Autodesk Inventor part; units mm, degrees
ref_plane "Work Plane1" through (0, 0, 0) normal (0, 0, 1) x (1, 0, 0)
ref_plane "Work Plane2" through (175.2488, -178.5172, -25.4) normal (0, 0, 1) x (0.3503, -0.9366, 0)
ref_plane "YZ Plane" through (0, 0, 0) normal (1, 0, 0) x (0, 1, 0)
ref_plane "Work Plane1" through (0, 0, 0) normal (0, 0, 1) x (1, 0, 0)
sketch "Sketch1" plane through (0, 0, 0) normal (0, 0, 1) x (1, 0, 0)
  circle A0 centre (0, 0) radius 12.7
  dimension "d0" = 25.4
extrude "Extrusion1" add sketch "Sketch1" against normal blind 50.8
sketch "Sketch2" plane through (0, 0, 0) normal (0, 0, 1) x (1, 0, 0)
  circle A0 centre (0, 0) radius 12.7
extrude "Extrusion2" add sketch "Sketch2" along normal blind 50.8
sketch "Sketch4" plane through (0, 0, 50.8) normal (0, 0, 1) x (1, 0, 0)
  circle A0 centre (0, 0) radius 38.1
  dimension "d6" = 76.2
extrude "Extrusion3" add sketch "Sketch4" along normal blind 25.4
ref_plane "Work Plane2" through (175.2488, -178.5172, -25.4) normal (0, 0, 1) x (0.3503, -0.9366, 0)
properties part number "clutch02-releaseMechanism" material "PET Plastic"
Here's how the part is built. I have some questions about the finished solid (model axes, mm). A direction names the side the tool comes from. Coordinates: 2 decimals unless noted, no trailing zeros. Write each loop counter-clockwise with the first axis right and the second up, starting at its lowest first coordinate (ties: lowest second). Pieces come first, ordered by that corner, then holes. Notation, with made-up numbers: M 74.25,50.5 L 90.25,50.5 A22 cw 90.25,75.5 Z; hole C 26.25,21 d9. An arc over 180 degrees is marked long. Answer as CSV lines item,"result". Start each with the question number.
Q1. Suppose I cut it at C-C, the plane z = -23.5. List the corners of the cut face in (x, y) for me, then the cut area to 3 significant figures.
Q2. Will these pins go through, and if not, where does the flat tip stop? pin 1 Ø2 at (y, z) = (-7, 5.5) entering from -X; pin 2 Ø12 at (x, y) = (30, 16.5) entering from -Z; pin 3 Ø5 at (x, z) = (7, 56) entering from +Y.
Q3. Suppose I cut it at D-D, the plane x = 32. List the corners of the cut face in (y, z) for me.
Q4. Suppose I cut it at A-A, the plane y = 0. List the corners of the cut face in (x, z) for me, then the cut area to 3 significant figures.
Q5. I need wall thicknesses on probe 1 along Z at (x, y) = (7, 27.5); probe 2 along X at (y, z) = (-10, -1.5); probe 3 along X at (y, z) = (16.5, 54). Which ranges of each line are inside material? Lowest first, please. Write a range as [from, to].
Q6. For faces 1 (the flat face through (0, 0, -50.8)), 2 (the cylindrical face through (-2.75, -12.4, 0.71)), which set-ups out of +Z, -Z, +X, -X, +Y, -Y let a thin tool reach every point of the face, with its end or its side?
Entries:
1,outline,"C 0,0 d25.4"
1,area,"507 mm²"
2,pin 1,"stops at x = -11.19"
2,pin 2,"stops at z = 50.8"
2,pin 3,"stops at y = 37.83"
3,outline,"M -20.68,50.8 L 20.68,50.8 L 20.68,76.2 L -20.68,76.2 Z"
4,outline,"M -38.1,50.8 L -12.7,50.8 L -12.7,-50.8 L 12.7,-50.8 L 12.7,50.8 L 38.1,50.8 L 38.1,76.2 L -38.1,76.2 Z"
4,area,"4,520 mm²"
5,probe 1,"z = [50.8, 76.2]"
5,probe 2,"x = [-7.83, 7.83]"
5,probe 3,"x = [-34.34, 34.34]"
6,face 1,"-Z, +X, -X, +Y, -Y"
6,face 2,"-Z"
